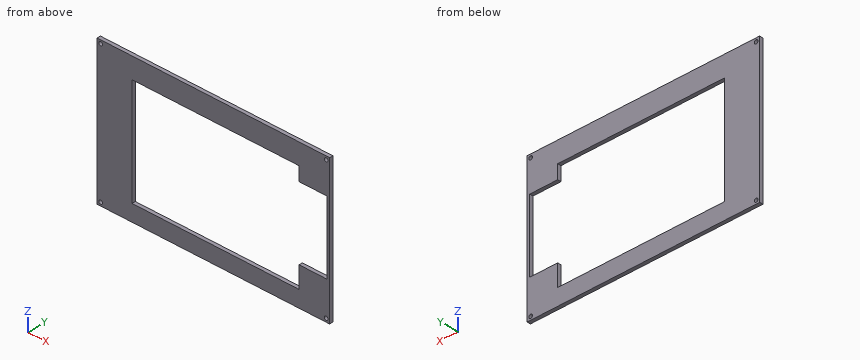
```python
from build123d import *

# Parameters (mm, degrees)
SKETCH_1_W      = 133
SKETCH_1_H      = 84
SKETCH_1_R      = 1.05
EXTRUDE_1_DEPTH = 2


with BuildPart() as part:
    # 草图1 → 凸台-拉伸1 (new body)
    with BuildSketch(Plane(origin=(0, 0, 0), x_dir=(1, 0, 0), z_dir=(0, 1, 0))):
        with Locations((66.5, -42)):
            Rectangle(SKETCH_1_W, SKETCH_1_H)
        with Locations(Location((2, -82, 0), (0, 0, 270))):
            Circle(SKETCH_1_R, mode=Mode.SUBTRACT)
        with Locations(Location((131, -82, 0), (0, 0, 270))):
            Circle(SKETCH_1_R, mode=Mode.SUBTRACT)
        with Locations(Location((2, -2, 0), (0, 0, 270))):
            Circle(SKETCH_1_R, mode=Mode.SUBTRACT)
        Polygon((20, -72), (20, -9.5), (115.5, -9.5), (115.5, -21.95), (131.5, -21.95), (131.5, -63.95), (115.5, -63.95), (115.5, -72), align=None, mode=Mode.SUBTRACT)
        with Locations(Location((131, -2, 0), (0, 0, 270))):
            Circle(SKETCH_1_R, mode=Mode.SUBTRACT)
    extrude(amount=EXTRUDE_1_DEPTH)


solid = part.part
```
Check sheet for the modelled part. Datum: model origin and axes. Units: mm. Coordinates: 2 decimals unless noted, no trailing zeros. Loops run counter-clockwise (first coordinate to the right, second up) from the corner with the lowest first, then second, coordinate; pieces in that order, holes last. Notation, with made-up numbers: M -7.5,45.5 L 35.5,45.5 A36 cw 35.5,79.5 Z; hole C 78.25,4 d8. An arc over 180 degrees is marked long. Answer as a JSON object with one key per item and string values.
1. Sectioned sample at B-B on y = 0.5. Record the cut outline in (x, z).
Outcome:
{"outline": "M 0,0 L 133,0 L 133,84 L 0,84 Z; hole C 2,2 d2.1; hole C 2,82 d2.1; hole M 20,9.5 L 115.5,9.5 L 115.5,21.95 L 131.5,21.95 L 131.5,63.95 L 115.5,63.95 L 115.5,72 L 20,72 Z; hole C 131,2 d2.1; hole C 131,82 d2.1"}
2. Sectioned sample at A-A on z = 35.5. Record the cut outline in (x, y), and give its area (3 significant figures).
Outcome:
{"outline": "M 0,0 L 20,0 L 20,2 L 0,2 Z; M 131.5,0 L 133,0 L 133,2 L 131.5,2 Z", "area": "43.0 mm²"}
3. Scan lines: L1, parallel to X at y = 0.6, z = 82; L2, parallel to Z at x = 131, y = 0.75; L3, parallel to Z at x = 71, y = 1.65. Record each from-to range of solid material in increasing order. Write a range as from..to.
Outcome:
{"L1": "0..0.95, 3.05..129.95, 132.05..133", "L2": "0..0.95, 3.05..21.95, 63.95..80.95, 83.05..84", "L3": "0..9.5, 72..84"}
4. Sectioned sample at C-C on x = 84.5. Record the cut outline in (y, z).
Outcome:
{"outline": "M 0,0 L 2,0 L 2,9.5 L 0,9.5 Z; M 0,72 L 2,72 L 2,84 L 0,84 Z"}
